```python
from build123d import *

# Parameters (mm, degrees)
F0_W          = 62.132306397
F0_H          = 98.6692346632
F1_DEPTH      = 25.4
F2_W          = 53.3400010318
F2_H          = 16.0215389915
F3_DEPTH      = 159.004
F3_DEPTH_BACK = 35.814
F4_R          = 5.08


with BuildPart() as f1:
    # F0 (on Top) → F1 (new body)
    with BuildSketch(Plane.XY):
        with Locations((1.5630759299, -9.1830771416)):
            Rectangle(F0_W, F0_H)
    extrude(amount=F1_DEPTH)

    # F2 (on Front) → F3 (cut, two sides)
    with BuildSketch(Plane.XZ) as f3_sk:
        with Locations((2.6376927271, 12.7976925578)):
            Rectangle(F2_W, F2_H)
    extrude(amount=-F3_DEPTH, mode=Mode.SUBTRACT)
    extrude(f3_sk.sketch, amount=F3_DEPTH_BACK, mode=Mode.SUBTRACT)

    # F4
    f4_edges = [f1.edges().sort_by_distance(p)[0] for p in [
        (32.629229, -9.183077, 25.4),
        (-29.503077, -9.183077, 25.4),
        (-29.503077, -9.183077, 0),
        (32.629229, -9.183077, 0),
    ]]
    fillet(f4_edges, radius=F4_R)


solid = f1.part
```
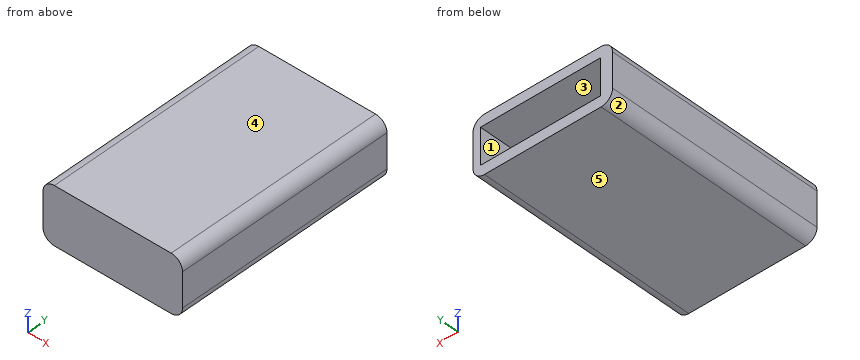
CAD build for the part. Positions are in the model's coordinates, mm. Face numbers are marked on the shaded views. A direction names the side the tool comes from. Round coordinates to 2 decimals unless told otherwise and drop trailing zeros. Order: outer loops, then holes, each group sorted by start corner. A loop starts at its lowest first (then second) coordinate and runs counter-clockwise, first axis right, second up.
Q1. Slice it at B-B (x = 24). Write the cut outline in (y, z), and give its area (3 significant figures).
Q2. Which spindle directions (+Z, -Z, +X, -X, +Y, -Y) get a long thin tool onto all of the face, cutting with end or side? Do the marked faces 1 and 2. Say none if no direction does.
Q3. Wall check: L1, parallel to X at y = 21, z = 13; L2, parallel to Z at x = 19.5, y = 4.5; L3, parallel to X at y = -48, z = 5. Give the ranges that are in metal, low to high.
Q4. Two-plate mould, pull along Z, no slides. Class the marked faces 3, 4 and 5: pulls with the +Z half, pulls with the -Z half, needs draft (parallel to the pull), parting line crosses it, or undercut.
Q5. Drop a flat-ended pin along its axis: pin 1 (6 mm diameter, centred on x = 14, z = 8.5, fed in from +Y). Give the stop position or say it passes through.
Q6. Slice it at A-A (y = 28.5). Write the cut outline in (x, z), and give its area (3 significant figures).
Q7. Slice it at C-C (z = 15.5). Write the cut outline in (x, y), and give its area (3 significant figures).
Q8. Slice it at D-D (z = 2). Write the cut outline in (x, y).
Results below:
1. outline: (-58.52, 0) - (40.15, 0) - (40.15, 4.79) - (-35.81, 4.79) - (-35.81, 20.81) - (40.15, 20.81) - (40.15, 25.4) - (-58.52, 25.4) - close
1. area: 1,290 mm2
2. face 1: +Y
2. face 2: -Z, -X, +Y, -Y
3. L1: x = -29.5 to -24.03, 29.31 to 32.63
3. L2: z = 0 to 4.79, 20.81 to 25.4
3. L3: x = -29.5 to 32.63
4. face 3: undercut
4. face 4: pulls with the +Z half
4. face 5: pulls with the -Z half
5. pin 1: stops at y = -35.81
6. outline: (-29.5, 5.08) arc R5.08 ccw to (-24.42, 0) - (27.55, 0) arc R5.08 ccw to (32.63, 5.08) - (32.63, 20.32) arc R5.08 ccw to (27.55, 25.4) - (-24.42, 25.4) arc R5.08 ccw to (-29.5, 20.32) - close; hole (-24.03, 4.79) - (29.31, 4.79) - (29.31, 20.81) - (-24.03, 20.81) - close
6. area: 701 mm2
7. outline: (-29.5, -58.52) - (32.63, -58.52) - (32.63, 40.15) - (29.31, 40.15) - (29.31, -35.81) - (-24.03, -35.81) - (-24.03, 40.15) - (-29.5, 40.15) - close
7. area: 2,080 mm2
8. outline: (-28.46, -58.52) - (31.59, -58.52) - (31.59, 40.15) - (-28.46, 40.15) - close
